Input: part model. Units: mm. Frame: model coordinates. Face numbers are marked on the shaded views. A direction names the side the tool comes from. Coordinates: 2 decimals unless noted, no trailing zeros. Write each loop counter-clockwise with the first axis right and the second up, starting at its lowest first coordinate (ties: lowest second). Pieces come first, ordered by that corner, then holes. Notation, with made-up numbers: (33, 84.25) - (78, 84.25) arc R26 ccw to (78, 122.25) - close; hole circle Ø8 at (50, 88.25). An arc over 180 degrees is marked (long way). Put each result on its own line as item: value. Start each with the question number.
1. Pin query (flat end, axial travel): pin 1 (0.5 mm diameter, centred on x = 6.5, z = -23.5, fed in from +Y); pin 2 (2.5 mm diameter, centred on x = 2.54, z = -2.54, fed in from -Y); pin 3 (4 mm diameter, centred on x = 21.5, y = -1.5, fed in from -Z); pin 4 (6 mm diameter, centred on x = 45, z = -20, fed in from -Y). Return the tip coordinate at first contact, or that it passes through.
2. Cut plane A-A, the plane z = -15. Return loops of the section in (x, y), and give its area (3 significant figures).
3. Cut plane B-B, the plane x = 19. Return loops of the section in (y, z), and give its area (3 significant figures).
4. Line query: line 1 (X direction, y = 1.1, z = -2.54); line 2 (Y direction, x = 53, z = -20); line 3 (Y direction, x = 14, z = -9). Output: solid intervals per line, ascending.
5. Cut plane C-C, the plane z = -25.5. Return loops of the section in (x, y), and give its area (3 significant figures).
6. Pull-direction query (X, two-part tool) for the marked faces 3 and 4; classes: released by +X, released by -X, zero draft, split by the parting line, or undercut.
7. Access query for the marked faces 1 and 2. Directions: +Z, -Z, +X, -X, +Y, -Y. A direction counts if a zero-diameter tool reaches every point of the face in a straight line with its end or side. Return the directions, or none.
from build123d import *

# Parameters (mm, degrees)
BOSS_EXTRUDE1_DEPTH = 1.5875
BOSS_EXTRUDE2_DEPTH = 2.8321
SKETCH3_W           = 1.778
SKETCH3_H           = 28.8036
BOSS_EXTRUDE3_DEPTH = 1.8161
SKETCH4_R           = 1.016
CUT_EXTRUDE1_DEPTH  = 66.623161235
SKETCH5_W           = 2.54
SKETCH5_H           = 25.4
BOSS_EXTRUDE4_DEPTH = 2.6289
SKETCH6_W           = 16.5608
SKETCH6_H           = 14.097
BOSS_EXTRUDE5_DEPTH = 1.8796


with BuildPart() as part:
    # Sketch1 → Boss-Extrude1 (new body)
    with BuildSketch(Plane(origin=(0, 0, 0), x_dir=(1, 0, 0), z_dir=(0, 1, 0))):
        with BuildLine():
            Line((2.54, 0), (53.34, 0))
            ThreePointArc((53.34, 0), (55.136051224, 0.743948776), (55.88, 2.54))
            Line((55.88, 2.54), (55.88, 31.75))
            ThreePointArc((55.88, 31.75), (55.136051224, 33.546051224), (53.34, 34.29))
            Line((53.34, 34.29), (2.54, 34.29))
            ThreePointArc((2.54, 34.29), (0.743948776, 33.546051224), (0, 31.75))
            Line((0, 31.75), (0, 2.54))
            ThreePointArc((0, 2.54), (0.743948776, 0.743948776), (2.54, 0))
        make_face()
    extrude(amount=BOSS_EXTRUDE1_DEPTH)

    # Sketch2 → Boss-Extrude2 (add)
    with BuildSketch(Plane(origin=(0, 1.5875, 0), x_dir=(1, 0, 0), z_dir=(0, 1, 0))):
        Polygon((50.292, 34.29), (3.7846, 34.29), (3.7846, 31.5468), (7.2009, 31.5468), (7.2009, 2.7432), (3.7846, 2.7432), (3.7846, 0), (50.292, 0), align=None)
    extrude(amount=BOSS_EXTRUDE2_DEPTH)

    # Sketch3 → Boss-Extrude3 (add)
    with BuildSketch(Plane(origin=(0, 1.5875, 0), x_dir=(1, 0, 0), z_dir=(0, 1, 0))):
        with Locations((6.3119, 17.145)):
            Rectangle(SKETCH3_W, SKETCH3_H)
    extrude(amount=BOSS_EXTRUDE3_DEPTH)

    # Sketch4 → Cut-Extrude1 (cut, through all)
    with BuildSketch(Plane(origin=(0, 1.5875, 0), x_dir=(1, 0, 0), z_dir=(0, 1, 0))):
        with Locations(Location((2.54, 31.75, 0), (0, 0, 270))):
            Circle(SKETCH4_R)
        with Locations(Location((2.54, 2.54, 0), (0, 0, 270))):
            Circle(SKETCH4_R)
        with Locations(Location((53.34, 31.75, 0), (0, 0, 270))):
            Circle(SKETCH4_R)
        with Locations(Location((53.34, 2.54, 0), (0, 0, 270))):
            Circle(SKETCH4_R)
    extrude(amount=-CUT_EXTRUDE1_DEPTH, mode=Mode.SUBTRACT)

    # Sketch5 → Boss-Extrude4 (add)
    with BuildSketch(Plane.XZ):
        with Locations((2.54, -17.145)):
            Rectangle(SKETCH5_W, SKETCH5_H)
    extrude(amount=BOSS_EXTRUDE4_DEPTH)

    # Sketch6 → Boss-Extrude5 (add)
    with BuildSketch(Plane.XZ):
        with Locations((47.5996, -17.145)):
            Rectangle(SKETCH6_W, SKETCH6_H)
    extrude(amount=BOSS_EXTRUDE5_DEPTH)


solid = part.part
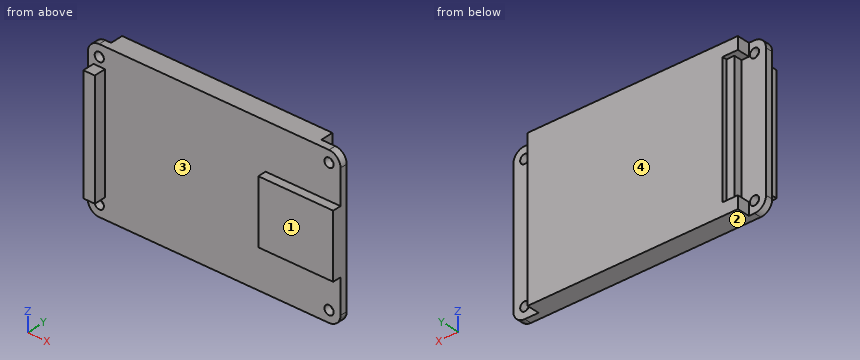
Report:
1. pin 1: stops at y = 3.4
1. pin 2: stops at y = 0
1. pin 3: stops at z = -34.29
1. pin 4: stops at y = -1.88
2. outline: (0, 0) - (1.27, 0) - (1.27, -2.63) - (3.81, -2.63) - (3.81, 0) - (39.32, 0) - (39.32, -1.88) - (55.88, -1.88) - (55.88, 1.59) - (50.29, 1.59) - (50.29, 4.42) - (7.2, 4.42) - (7.2, 3.4) - (5.42, 3.4) - (5.42, 1.59) - (0, 1.59) - close
2. area: 252 mm^2
3. outline: (0, -34.29) - (4.42, -34.29) - (4.42, 0) - (0, 0) - close
3. area: 152 mm^2
4. line 1: x = 0 to 1.52, 3.56 to 52.32, 54.36 to 55.88
4. line 2: y = -1.88 to 1.59
4. line 3: y = 0 to 4.42
5. outline: (0, 0) - (1.27, 0) - (1.27, -2.63) - (3.81, -2.63) - (3.81, 0) - (55.88, 0) - (55.88, 1.59) - (50.29, 1.59) - (50.29, 4.42) - (7.2, 4.42) - (7.2, 3.4) - (5.42, 3.4) - (5.42, 1.59) - (0, 1.59) - close
5. area: 221 mm^2
6. face 3: undercut
6. face 4: zero draft
7. face 1: +Z, -Z, +X, -Y
7. face 2: -Z, +X, -X, +Y, -Y
